Autodesk Inventor part; units mm, degrees
ref_plane "YZ Plane" through (0, 0, 0) normal (1, 0, 0) x (0, 1, 0)
ref_plane "XZ Plane" through (0, 0, 0) normal (0, 1, 0) x (-1, 0, 0)
ref_plane "XY Plane" through (0, 0, 0) normal (0, 0, 1) x (1, 0, 0)
sketch "Sketch1" plane through (0, 0, 0) normal (0, 0, 1) x (1, 0, 0)
  circle A0 centre (0, 0) radius 41.148
  dimension "d0" = 82.296
extrude "Extrusion1" add sketch "Sketch1" against normal blind 95.504
sketch "Sketch2" plane through (0, 0, 0) normal (0, 0, 1) x (1, 0, 0)
  circle A0 centre (0, 0) radius 22.098
  dimension "d3" = 44.196
extrude "Extrusion2" cut sketch "Sketch2" against normal blind 95.504
sketch "Sketch3" plane through (0, 0, -95.504) normal (0, 0, -1) x (-1, 0, 0)
  circle A0 centre (0, 0) radius 41.148
  circle A1 centre (0, 0) radius 28.575
  dimension "d6" = 57.15
extrude "Extrusion3" cut sketch "Sketch3" against normal blind 24.13
sketch "Sketch4" plane through (0, 0, 0) normal (0, 0, 1) x (1, 0, 0)
  circle A0 centre (0, 0) radius 22.098
  circle A1 centre (0, 0) radius 28.575
  dimension "d9" = 57.15
extrude "Extrusion4" cut sketch "Sketch4" against normal blind 6.35
sketch "Sketch5" plane through (0, 0, 0) normal (0, 0, 1) x (1, 0, 0)
  circle A0 centre (0, 0) radius 41.148
  circle A1 centre (0, 0) radius 31.75
  dimension "d12" = 63.5
extrude "Extrusion5" cut sketch "Sketch5" against normal blind 65.024
sketch "Sketch6" plane through (0, 0, 0) normal (0, 0, 1) x (1, 0, 0)
  circle A0 centre (0, 0) radius 31.75
  circle A1 centre (0, 0) radius 41.148
extrude "Extrusion6" add sketch "Sketch6" against normal blind 12.7
sketch "Sketch7" plane through (0, 0, 0) normal (0, 0, 1) x (1, 0, 0)
  circle A0 centre (0, 36.449) radius 2.3813
  circle A1 centre (-31.5658, 18.2245) radius 2.3813
  circle A2 centre (-31.5658, -18.2245) radius 2.3813
  circle A3 centre (0, -36.449) radius 2.3813
  circle A4 centre (31.5658, -18.2245) radius 2.3813
  circle A5 centre (31.5658, 18.2245) radius 2.3813
  point P0 (0, 0)
  dimension "d17" = 4.7625
  dimension "d20" = 360
extrude "Extrusion7" cut sketch "Sketch7" against normal blind 152.4
properties part number "PostComb4_4"
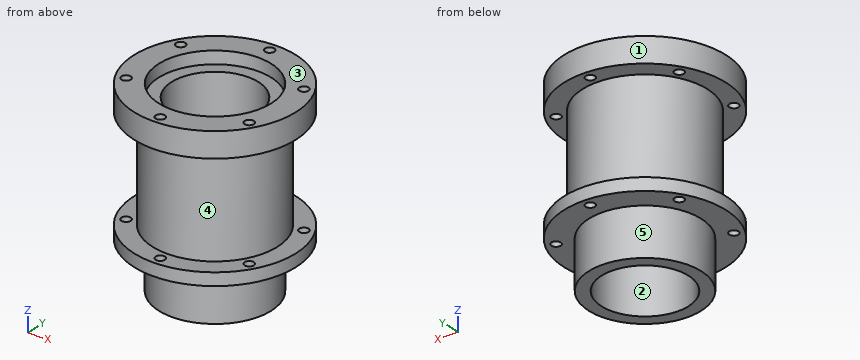
For this review, take the finished solid that the model builds, in its own axes (mm). Face numbers are marked on the shaded views. A direction names the side the tool comes from. Coordinates: 2 decimals unless noted, no trailing zeros. Write each loop counter-clockwise with the first axis right and the second up, starting at its lowest first coordinate (ties: lowest second). Pieces come first, ordered by that corner, then holes. Notation, with made-up numbers: (-21, 66) - (-4, 66) arc R36 cw to (-4, 100) - close; hole circle Ø4 at (76, 21.25). An arc over 180 degrees is marked (long way). Answer in a Markdown table with one row per item. Add a question column.
Q1. We need section A-A, the plane y = 0. State the section outline as (x, z) points (3 decimals), and give its area (3 significant figures).
Q2. Tool access review of the marked faces 4 and 5: name each direction out of +Z, -Z, +X, -X, +Y, -Y from which nothing blocks a thin tool from reaching the whole face with its end or side.
Q3. We need section D-D, the plane x = -8.5. State the section outline as (y, z) points, and give its area (3 significant figures).
Q4. We need section B-B, the plane x = 0. Count the separate pieces of the cut face and the enclosed holes in it, and give its area (3 significant figures).
Q5. Draft analysis for pull direction Y (two halves, no side actions). For the marked faces 1, 2 and 3, state which applies: +Y half, -Y half, draft (parallel to the pull), parting line (faces both ways), or undercut.
Q6. For P1, Ø5.5, axis at x = 0, y = -36.449, coming from the -Z side; P2, Ø10, axis at y = 3.5, z = -83.5, coming from the +X side (3 decimals); P3, Ø3, axis at x = -2.5, z = -31, coming from the +Y side, all flat-tipped, find the tip position at first contact; note any pin that passes through.
Q7. For probe 1 along Z at (x, y) = (34, 3); probe 2 along Z at (x, y) = (23, 13); probe 3 along Y at (x, z) = (30, -67), list the stretches that pass through material, from the lowest coordinate up.
Q8. We need section C-C, the plane z = -73. State the section outline as (x, y) points (3 decimals).
Answer list:
| question | item | result |
|---|---|---|
| 1 | outline | (-41.148, -71.374) - (-28.575, -71.374) - (-28.575, -95.504) - (-22.098, -95.504) - (-22.098, -6.35) - (-28.575, -6.35) - (-28.575, 0) - (-41.148, 0) - (-41.148, -12.7) - (-31.75, -12.7) - (-31.75, -65.024) - (-41.148, -65.024) - close; (22.098, -95.504) - (28.575, -95.504) - (28.575, -71.374) - (41.148, -71.374) - (41.148, -65.024) - (31.75, -65.024) - (31.75, -12.7) - (41.148, -12.7) - (41.148, 0) - (28.575, 0) - (28.575, -6.35) - (22.098, -6.35) - close |
| 1 | area | 1,970 mm2 |
| 2 | face 4 | none |
| 2 | face 5 | -Z |
| 3 | outline | (-40.26, -71.37) - (-27.28, -71.37) - (-27.28, -95.5) - (-20.4, -95.5) - (-20.4, -6.35) - (-27.28, -6.35) - (-27.28, 0) - (-40.26, 0) - (-40.26, -12.7) - (-30.59, -12.7) - (-30.59, -65.02) - (-40.26, -65.02) - close; (20.4, -95.5) - (27.28, -95.5) - (27.28, -71.37) - (40.26, -71.37) - (40.26, -65.02) - (30.59, -65.02) - (30.59, -12.7) - (40.26, -12.7) - (40.26, 0) - (27.28, 0) - (27.28, -6.35) - (20.4, -6.35) - close |
| 3 | area | 2,070 mm2 |
| 4 | separate pieces | 6 |
| 4 | enclosed holes | 0 |
| 4 | area | 1,780 mm2 |
| 5 | face 1 | parting line |
| 5 | face 2 | undercut |
| 5 | face 3 | draft |
| 6 | P1 | stops at z = -71.37 |
| 6 | P2 | stops at x = 28.575 |
| 6 | P3 | stops at y = 31.73 |
| 7 | probe 1 | z = -71.37 to -65.02, -12.7 to 0 |
| 7 | probe 2 | z = -95.5 to -6.35 |
| 7 | probe 3 | y = -28.16 to -20.02, -16.43 to 16.43, 20.02 to 28.16 |
| 8 | outline | circle Ø57.15 at (0, 0); hole circle Ø44.196 at (0, 0) |
